Can you work these out from the model? Positions are in its coordinate system, mm. Face numbers are marked on the shaded views. Round coordinates to 2 decimals unless told otherwise and drop trailing zeros. Write each loop counter-clockwise with the first axis right and the second up, starting at its lowest first coordinate (ties: lowest second). Pieces come first, ordered by that corner, then holes. Notation, with made-up numbers: M 6.25,1 L 64.25,1 A31 ccw 64.25,37 Z; hole C -11,-13 d5. An arc over 180 degrees is marked long. Answer in a Markdown table with one row per item. Add a question column.
(1) If we mould it in two halves opening along X, with no side actions, what happens to the marked faces 1, 2, 3 and 4? For each: released by +X, released by -X, zero draft, split by the parting line, or undercut.
(2) Suppose I cut it at D-D, the plane z = 8.25. Write out the boundary of the cut face in (x, y), then the cut area to 3 significant figures.
(3) If I drill on probe 1 along Y at (x, z) = (0, 2.5); probe 2 along Y at (x, z) = (-5.5, 5.75); probe 3 along Y at (x, z) = (0.75, 4.5), over which ranges is the centre line in solid material (lowest first)?
(4) Suppose I cut it at A-A, the plane y = 0. Write out the boundary of the cut face in (x, z).
(5) Suppose I cut it at C-C, the plane z = 4.5. Write out the boundary of the cut face in (x, y), then the cut area to 3 significant figures.
(6) Suppose I cut it at B-B, the plane x = 0. Write out the boundary of the cut face in (y, z), then the cut area to 3 significant figures.
from build123d import *

# Parameters (mm, degrees)
SKETCH1_W           = 13
SKETCH1_H           = 20
SKETCH1_R           = 4
BOSS_EXTRUDE1_DEPTH = 10
SKETCH2_R           = 1
CUT_EXTRUDE1_DEPTH  = 20.209372712


with BuildPart() as part:
    # Sketch1 → Boss-Extrude1 (new body)
    with BuildSketch(Plane.XY):
        Rectangle(SKETCH1_W, SKETCH1_H)
        Circle(SKETCH1_R, mode=Mode.SUBTRACT)
    extrude(amount=BOSS_EXTRUDE1_DEPTH)

    # Sketch2 → Cut-Extrude1 (cut, through all)
    with BuildSketch(Plane(origin=(6.5, 0, 0), x_dir=(0, 0, -1), z_dir=(1, 0, 0))):
        with Locations((-5.057573934, 7.718180526)):
            Circle(SKETCH2_R)
    cut_extrude1 = extrude(amount=-CUT_EXTRUDE1_DEPTH, mode=Mode.SUBTRACT)

    # Mirror1: Cut-Extrude1 across plane
    add(cut_extrude1.mirror(Plane.ZX), mode=Mode.SUBTRACT)


solid = part.part
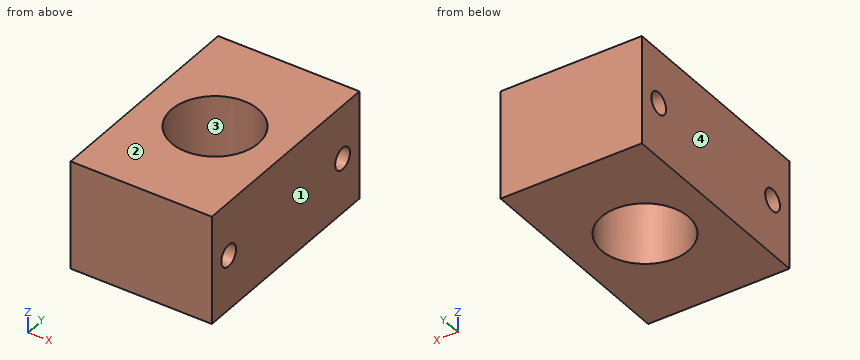
Calculated:
| question | item | result |
|---|---|---|
| 1 | face 1 | released by +X |
| 1 | face 2 | zero draft |
| 1 | face 3 | undercut |
| 1 | face 4 | released by -X |
| 2 | outline | M -6.5,-10 L 6.5,-10 L 6.5,10 L -6.5,10 Z; hole C 0,0 d8 |
| 2 | area | 210 mm² |
| 3 | probe 1 | -10 to -4, 4 to 10 |
| 3 | probe 2 | -10 to -8.44, -7 to 7, 8.44 to 10 |
| 3 | probe 3 | -10 to -8.55, -6.89 to -3.93, 3.93 to 6.89, 8.55 to 10 |
| 4 | outline | M -6.5,0 L -4,0 L -4,10 L -6.5,10 Z; M 4,0 L 6.5,0 L 6.5,10 L 4,10 Z |
| 5 | outline | M -6.5,-10 L 6.5,-10 L 6.5,-8.55 L -6.5,-8.55 Z; M -6.5,-6.89 L 6.5,-6.89 L 6.5,6.89 L -6.5,6.89 Z; M -6.5,8.55 L 6.5,8.55 L 6.5,10 L -6.5,10 Z; hole C 0,0 d8 |
| 5 | area | 167 mm² |
| 6 | outline | M -10,0 L -4,0 L -4,10 L -10,10 Z; M 4,0 L 10,0 L 10,10 L 4,10 Z; hole C -7.72,5.06 d2; hole C 7.72,5.06 d2 |
| 6 | area | 114 mm² |
